Geometry check sheet. Reference: the model listing, model coordinates, mm. Face numbers are marked on the shaded views. A direction names the side the tool comes from. Round coordinates to 2 decimals unless told otherwise and drop trailing zeros. Write each loop counter-clockwise with the first axis right and the second up, starting at its lowest first coordinate (ties: lowest second). Pieces come first, ordered by that corner, then holes. Notation, with made-up numbers: (30, 2) -> (45, 2) arc R16 ccw to (45, 33) -> close; hole circle Ø11 at (31, 4.5). An arc over 180 degrees is marked (long way). One line per question, with ' | ' between items.
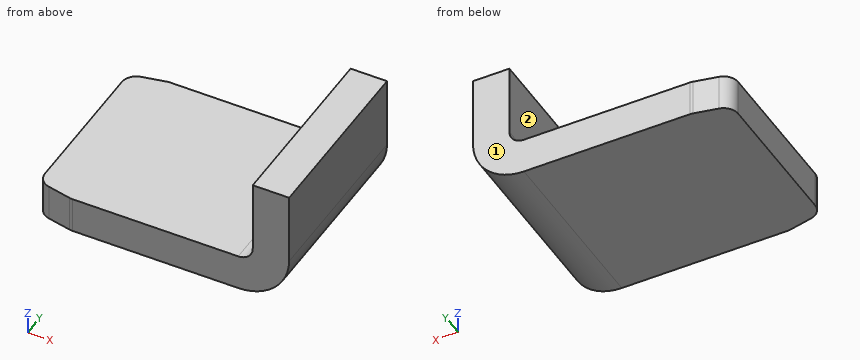
Autodesk Inventor part; units mm, degrees
ref_plane "YZ Plane" through (0, 0, 0) normal (1, 0, 0) x (0, 1, 0)
ref_plane "XZ Plane" through (0, 0, 0) normal (0, 1, 0) x (-1, 0, 0)
ref_plane "XY Plane" through (0, 0, 0) normal (0, 0, 1) x (1, 0, 0)
sketch "Sketch1" plane through (0, 0, 0) normal (0, 0, 1) x (1, 0, 0)
  line L0 (4.3681, -1.3047) -> (34.1579, -1.3047)
  line L1 (34.1579, -1.3047) -> (34.1579, 23.6953)
  line L2 (34.1579, 23.6953) -> (4.3681, 23.6953)
  line L3 (-0.8421, 21.0129) -> (-0.8421, 1.3776)
  line L4 (3.9523, 23.6516) -> (0.7421, 22.9692)
  line L5 (3.9523, -1.261) -> (0.7421, -0.5787)
  line L6 (4.1579, 23.6953) -> (4.1579, -1.3047) construction
  arc A0 (0.7421, 22.9692) -> (-0.8421, 21.0129) centre (1.1579, 21.0129) ccw
  arc A1 (-0.8421, 1.3776) -> (0.7421, -0.5787) centre (1.1579, 1.3776) ccw
  arc A2 (4.3681, 23.6953) -> (3.9523, 23.6516) centre (4.3681, 21.6953) ccw
  arc A3 (3.9523, -1.261) -> (4.3681, -1.3047) centre (4.3681, 0.6953) ccw
  point P0 (0, 0)
  point P1 (-0.8421, 22.6325)
  point P2 (-0.8421, -0.242)
  dimension "d3" = 12
  dimension "d4" = 25
  dimension "d5" = 12
  dimension "d7" = 35
  dimension "d8" = 5
  dimension "d20" = 2
extrude "Plate1" add sketch "Sketch1" along normal blind 5
sketch "Sketch2" plane through (29.1579, 23.6953, 0) normal (1, 0, 0) x (0, 1, 0)
  line L0 (-25, 0) -> (0, 0)
  line L1 (0, 0) -> (0, 17)
  line L2 (0, 17) -> (-25, 17)
  line L3 (-25, 17) -> (-25, 0)
edge flange "Flange1" height 12 angle 90 thickness 5 bend radius 2 thickness toward (1, 0, 0) relief tear relief width 5 relief depth 2.5 edges at (34.1579, 11.1953, 5) wall of the first edge with corners at (29.1579, -1.3047, 0) (29.1579, 23.6953, 0) (29.1579, 23.6953, 17) (29.1579, -1.3047, 17)
bend "Bend1"
corner "Corner1"
ref_plane "midtplan" through (4.3681, 11.1953, 5) normal (0, 1, 0) x (1, 0, 0)
equation "\"d3\" = d5"
equation "\"d9\" = Thickness"
equation "\"d10\" = BendReliefWidth"
equation "\"d11\" = BendReliefDepth"
equation "\"d12\" = MinimumRemnant"
equation "\"d13\" = TransitionRadius"
equation "\"d16\" = BendRadius"
equation "\"d17\" = CornerReliefSize"
equation "\"d18\" = GapSize"
equation "\"d19\" = JacobiRadiusSize"
equation "\"BendReliefWidth\" = Thickness"
equation "\"BendReliefDepth\" = 0.5 * Thickness"
equation "\"TransitionRadius\" = BendRadius"
equation "\"JacobiRadiusSize\" = BendRadius"
equation "\"GapSize\" = Thickness"
properties part number "hage" material "Steel"
(1) Sectioned sample at C-C on z = 14.5. Record the cut outline in (x, y).
Resolved:
outline: (29.16, -1.3) -> (34.16, -1.3) -> (34.16, 23.7) -> (29.16, 23.7) -> close
(2) Material ranges on line 1 (Z direction, x = 22.5, y = 3.75); line 2 (X direction, y = 13.25, z = 13.25); line 3 (Z direction, x = 32, y = 4.25), recorded low to high.
Resolved:
line 1: z = 0 to 5 | line 2: x = 29.16 to 34.16 | line 3: z = 1.94 to 17
(3) Access from +Z, -Z, +X, -X, +Y, -Y to the whole of each face (thin tool, end or side, straight path). Record for the marked faces 1 and 2.
Resolved:
face 1: +Z, -Z, +X, -X, +Y | face 2: +Z, -X, +Y, -Y
(4) Sectioned sample at B-B on x = 12.5. Record the cut outline in (y, z), then the cut area to 3 significant figures.
Resolved:
outline: (-1.3, 0) -> (23.7, 0) -> (23.7, 5) -> (-1.3, 5) -> close | area: 125 mm2
(5) Go/stop test with flat-tipped pins: pin 1 (8 mm diameter, centred on x = 15, z = 12, fed in from +Y); pin 2 (1.5 mm diameter, centred on x = 7.5, y = 19, fed in from -Z); pin 3 (3 mm diameter, centred on x = 17.5, y = 8.5, fed in from +Z); pin 4 (8 mm diameter, centred on y = 11, z = 12, fed in from -X). Record where each tip stops, or that it passes through.
Resolved:
pin 1: passes through | pin 2: stops at z = 0 | pin 3: stops at z = 5 | pin 4: stops at x = 29.16
(6) Sectioned sample at A-A on y = 18. Record the cut outline in (x, z).
Resolved:
outline: (-0.84, 0) -> (27.16, 0) arc R7 ccw to (34.16, 7) -> (34.16, 17) -> (29.16, 17) -> (29.16, 7) arc R2 cw to (27.16, 5) -> (-0.84, 5) -> close
(7) Sectioned sample at D-D on z = 4. Record the cut outline in (x, y).
Resolved:
outline: (-0.84, 1.38) arc R2 ccw to (0.74, -0.58) -> (3.95, -1.26) arc R2 ccw to (4.37, -1.3) -> (33.48, -1.3) -> (33.48, 23.7) -> (4.37, 23.7) arc R2 ccw to (3.95, 23.65) -> (0.74, 22.97) arc R2 ccw to (-0.84, 21.01) -> close
